from build123d import *

# Parameters (mm, degrees)
EXTRUDE_1_DEPTH          = 10
CUT_EXTRUDE_1_DEPTH      = 40.37003937
CUT_EXTRUDE_1_DEPTH_BACK = 40.37003937
SKETCH_2_R               = 1.5


with BuildPart() as part:
    # 草图1 → 凸台-拉伸1 (new body)
    with BuildSketch(Plane.XY):
        Polygon((-20, 0), (-10, 0), (-10, 10), (10, 10), (10, 0), (20, 0), (35, 0), (35, 5), (20, 5), (20, 15), (15, 15), (15, 20), (-15, 20), (-15, 15), (-20, 15), (-20, 5), (-35, 5), (-35, 0), align=None)
    extrude(amount=EXTRUDE_1_DEPTH)

    # 草图2 → 切除-拉伸1 (cut, two sides: drawn at the far end of the back side and taken through both)
    with BuildSketch(Plane(origin=(0, 5, 0), x_dir=(1, 0, 0), z_dir=(0, 1, 0)).offset(-CUT_EXTRUDE_1_DEPTH_BACK)):
        with Locations(Location((-27.5, -5, 0), (0, 0, 180))):
            Circle(SKETCH_2_R)
        with Locations(Location((27.5, -5, 0), (0, 0, 180))):
            Circle(SKETCH_2_R)
    extrude(amount=CUT_EXTRUDE_1_DEPTH + CUT_EXTRUDE_1_DEPTH_BACK, mode=Mode.SUBTRACT)


solid = part.part
The model under review builds one solid part; all positions refer to its coordinate system, in mm. A direction names the side the tool comes from. Give positions to 0.01 mm unless a question says otherwise; leave off trailing zeros. Loops run counter-clockwise (first coordinate to the right, second up) from the corner with the lowest first, then second, coordinate; pieces in that order, holes last. Notation, with made-up numbers: (50.25, 7) -> (62.25, 7) arc R9 ccw to (62.25, 16) -> close; hole circle Ø7 at (47.25, -8). An arc over 180 degrees is marked (long way). Put each result on its own line as item: value. Start each with the question number.
1. We need section B-B on y = 6.5. State the section outline as (x, z) points.
2. We need section D-D on z = 4.25. State the section outline as (x, y) points, then the cut area to 3 significant figures.
3. We need section C-C on x = 27.5. State the section outline as (y, z) points, then the cut area to 3 significant figures.
4. For faces 1 (the face through (-25.7, 5, 4.9)), 2 (the face through (29.3, 5, 4.9)), 3 (the face through (10, 5, 5)), 4 (the face through (-35, 3, 5)), 5 (the face through (0, 12, 10)), list the 3-axis set-ups (+Z, -Z, +X, -X, +Y, -Y) from which the entire face can be reached by the end or side of a thin tool; tool diameter is ignored.
5. Clearance check with flat-ended pins moving along their axes: P1, Ø5, axis at y = 11, z = 3.5, coming from the +X side; P2, Ø5.5, axis at x = 18, z = 4.5, coming from the +Y side; P3, Ø2.5, axis at y = 17.5, z = 7.5, coming from the +X side. State where each tip first meets the part, or that it passes through.
6. Mouldability with a two-part tool opening along X and no side actions: class faces 6 (the face through (-17, 15, 5)), 7 (the face through (-26, 2, 5)), 8 (the face through (35, 2, 5)) as released by +X, released by -X, zero draft, split by the parting line, or undercut.
7. We need section A-A on y = 3. State the section outline as (x, z) points.
8. Wall thickness on probe 1 along X at (y, z) = (3.1, 5); probe 2 along X at (y, z) = (9.5, 4.5); probe 3 along X at (y, z) = (2.25, 0.75): over which ranges is each line inside the solid? List them lowest first.
Determined:
1. outline: (-20, 0) -> (-10, 0) -> (-10, 10) -> (-20, 10) -> close; (10, 0) -> (20, 0) -> (20, 10) -> (10, 10) -> close
2. outline: (-35, 0) -> (-28.8, 0) -> (-28.8, 5) -> (-35, 5) -> close; (-26.2, 0) -> (-10, 0) -> (-10, 10) -> (10, 10) -> (10, 0) -> (26.2, 0) -> (26.2, 5) -> (20, 5) -> (20, 15) -> (15, 15) -> (15, 20) -> (-15, 20) -> (-15, 15) -> (-20, 15) -> (-20, 5) -> (-26.2, 5) -> close; (28.8, 0) -> (35, 0) -> (35, 5) -> (28.8, 5) -> close
2. area: 674 mm^2
3. outline: (0, 0) -> (5, 0) -> (5, 3.5) -> (0, 3.5) -> close; (0, 6.5) -> (5, 6.5) -> (5, 10) -> (0, 10) -> close
3. area: 35.0 mm^2
4. face 1: +Z, -Z, -X, +Y
4. face 2: +Z, -Z, +X, +Y
4. face 3: +Z, -Z, -Y
4. face 4: +Z, -Z, -X, +Y, -Y
4. face 5: +Z, +X, -X, +Y, -Y
5. P1: x = 20
5. P2: y = 15
5. P3: x = 15
6. face 6: zero draft
6. face 7: undercut
6. face 8: released by +X
7. outline: (-35, 0) -> (-10, 0) -> (-10, 10) -> (-35, 10) -> close; (10, 0) -> (35, 0) -> (35, 10) -> (10, 10) -> close; hole circle Ø3 at (-27.5, 5); hole circle Ø3 at (27.5, 5)
8. probe 1: -35 to -29, -26 to -10, 10 to 26, 29 to 35
8. probe 2: -20 to -10, 10 to 20
8. probe 3: -35 to -10, 10 to 35
